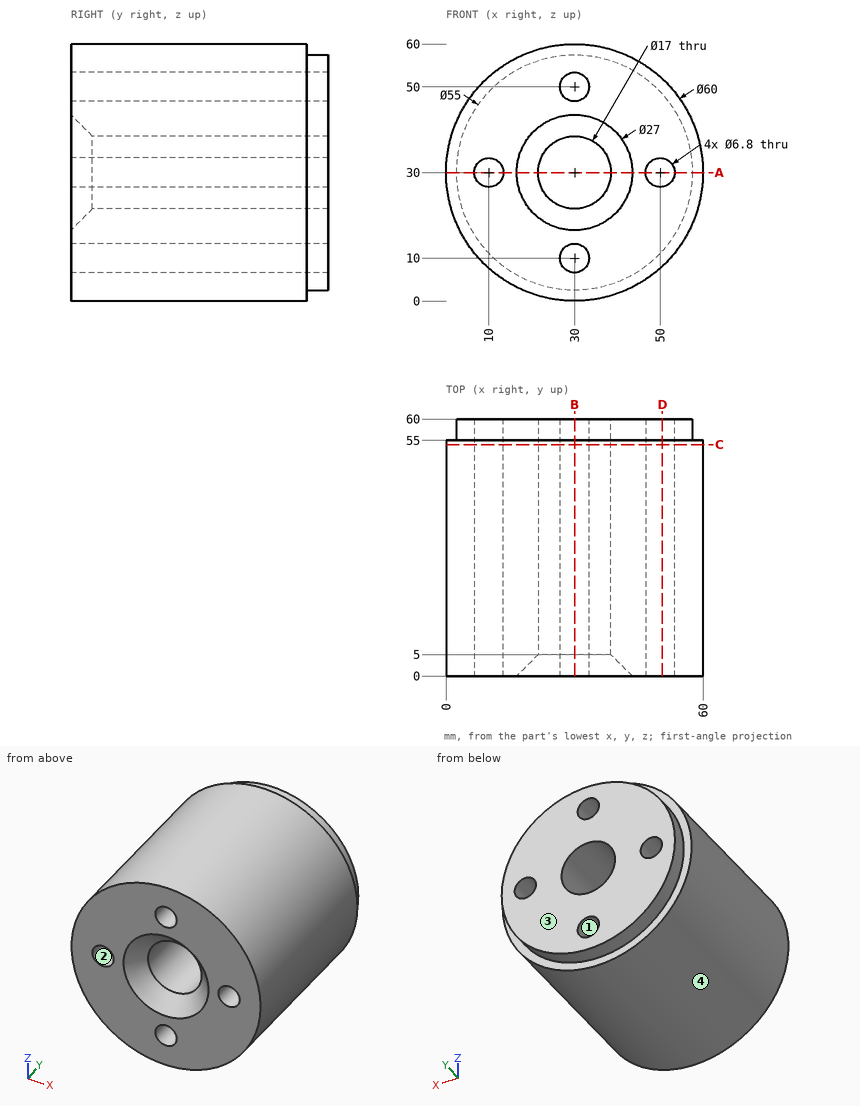
Design review of the part shown in the three views and the two pictorial views. Dimensions are in mm from the part's minimum x, y and z. Round coordinates to 2 decimals unless told otherwise and drop trailing zeros. Write each loop counter-clockwise with the first axis right and the second up, starting at its lowest first coordinate (ties: lowest second). Pieces come first, ordered by that corner, then holes.
Item 1: Consider section C-C on y = 54. Give the boundary of the cut face in (x, z), and give its area (3 significant figures).
Item 2: Consider section D-D on x = 50.5. Give the boundary of the cut face in (y, z).
Item 3: Consider section B-B on x = 30. Give the boundary of the cut face in (y, z), and give its area (3 significant figures).
Item 4: Consider section A-A on z = 30. Give the boundary of the cut face in (x, y), and give its area (3 significant figures).
Item 5: For pin 1 Ø9 at (x, z) = (50, 30) entering from +Y; pin 2 Ø1 at (x, y) = (42, 20) entering from -Z; pin 3 Ø8 at (y, z) = (34, 47.5) entering from +X; pin 4 Ø5 at (y, z) = (37, 8) entering from +X, all flat-tipped, find the tip position at first contact; note any pin that passes through.
Item 6: Wall thickness on L1, parallel to Z at x = 30, y = 30.5; L2, parallel to Z at x = 33, y = 8: over which ranges is each line inside the solid? List them lowest first.
Item 7: Draft analysis for pull direction X (two halves, no side actions). For the marked faces 1, 2, 3 and 4, state which applies: released by +X, released by -X, zero draft, split by the parting line, or undercut.
Check values:
1. outline: circle Ø60 at (30, 30); hole circle Ø6.8 at (10, 30); hole circle Ø17 at (30, 30); hole circle Ø6.8 at (30, 10); hole circle Ø6.8 at (30, 50); hole circle Ø6.8 at (50, 30)
1. area: 2,460 mm2
2. outline: (0, 8.1) - (55, 8.1) - (55, 11.67) - (60, 11.67) - (60, 26.64) - (0, 26.64) - close; (0, 33.36) - (60, 33.36) - (60, 48.33) - (55, 48.33) - (55, 51.9) - (0, 51.9) - close
3. outline: (0, 0) - (55, 0) - (55, 2.5) - (60, 2.5) - (60, 6.6) - (0, 6.6) - close; (0, 13.4) - (60, 13.4) - (60, 21.5) - (5, 21.5) - (0, 16.5) - close; (0, 43.5) - (5, 38.5) - (60, 38.5) - (60, 46.6) - (0, 46.6) - close; (0, 53.4) - (60, 53.4) - (60, 57.5) - (55, 57.5) - (55, 60) - (0, 60) - close
3. area: 1,710 mm2
4. outline: (0, 0) - (6.6, 0) - (6.6, 60) - (2.5, 60) - (2.5, 55) - (0, 55) - close; (13.4, 0) - (16.5, 0) - (21.5, 5) - (21.5, 60) - (13.4, 60) - close; (38.5, 5) - (43.5, 0) - (46.6, 0) - (46.6, 60) - (38.5, 60) - close; (53.4, 0) - (60, 0) - (60, 55) - (57.5, 55) - (57.5, 60) - (53.4, 60) - close
4. area: 1,710 mm2
5. pin 1: stops at y = 60
5. pin 2: stops at z = 2.29
5. pin 3: stops at x = 56.79
5. pin 4: stops at x = 52.8
6. L1: z = 0 to 6.6, 13.4 to 21.5, 38.5 to 46.6, 53.4 to 60
6. L2: z = 0.15 to 8.4, 11.6 to 22.05, 37.95 to 48.4, 51.6 to 59.85
7. face 1: undercut
7. face 2: undercut
7. face 3: zero draft
7. face 4: split by the parting line
